Check sheet for the modelled part. Datum: model origin and axes. Units: mm. Face numbers are marked on the shaded views. A direction names the side the tool comes from. Coordinates: 2 decimals unless noted, no trailing zeros. Loops run counter-clockwise (first coordinate to the right, second up) from the corner with the lowest first, then second, coordinate; pieces in that order, holes last. Notation, with made-up numbers: (8.5, 48) -> (44.5, 48) arc R31 ccw to (44.5, 76) -> close; hole circle Ø7 at (-30.5, -17). An arc over 180 degrees is marked (long way). Use CSV: the item, a comma, the result in double quotes.
```python
from build123d import *

# Parameters (mm, degrees)
BOSS_EXTRUDE1_START = 0.2
BOSS_EXTRUDE1_DEPTH = 1
BOSS_EXTRUDE2_DEPTH = 0.2


with BuildPart() as part:
    # Sketch1 → Boss-Extrude1 (new body)
    with BuildSketch(Plane.XY.offset(BOSS_EXTRUDE1_START)):
        Polygon((-2.65, 2.65), (2.65, 2.65), (2.65, -1.15), (1.15, -2.65), (-1.15, -2.65), (-2.65, -1.15), align=None)
    extrude(amount=BOSS_EXTRUDE1_DEPTH)

    # Sketch2 → Revolve1 (revolve)
    with BuildSketch(Plane(origin=(0, 0, 0), x_dir=(0, 0, -1), z_dir=(1, 0, 0)), mode=Mode.PRIVATE) as revolve1_sk:
        with BuildLine():
            Line((-6, 0), (-6, 2.5))
            Line((-6, 2.5), (-2.2, 2.5))
            ThreePointArc((-2.2, 2.5), (-1.8, 2.1), (-1.4, 2.5))
            Line((-1.4, 2.5), (-1.2, 2.5))
            Line((-1.2, 2.5), (-1.2, 0))
            Line((-1.2, 0), (-6, 0))
        make_face()
    revolve(revolve1_sk.sketch.rotate(Axis((0, 0, 0), (0, 0, 1)), 90), axis=Axis((0, 0, 0), (0, 0, 1)))

    # Sketch3 → Boss-Extrude2 (add)
    with BuildSketch(Plane.XY):
        with BuildLine():
            Line((0.4, -1.1), (0.4, -3))
            Line((0.4, -3), (-0.4, -3))
            Line((-0.4, -3), (-0.4, -1.1))
            ThreePointArc((-0.4, -1.1), (0, -0.7), (0.4, -1.1))
        make_face()
    boss_extrude2 = extrude(amount=BOSS_EXTRUDE2_DEPTH)

    # Mirror1: Boss-Extrude2 across plane
    add(boss_extrude2.mirror(Plane.ZX))


solid = part.part
```
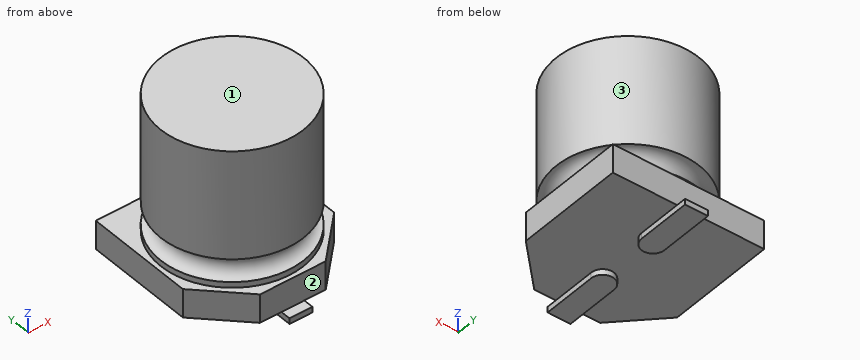
1) Cross-section at B-B on y = 0. Record the boundary of the cut face in (x, z).
Answer below:
outline,"(-2.65, 0.2) -> (2.65, 0.2) -> (2.65, 1.2) -> (2.5, 1.2) -> (2.5, 1.4) arc R0.4 cw to (2.5, 2.2) -> (2.5, 6) -> (-2.5, 6) -> (-2.5, 2.2) arc R0.4 cw to (-2.5, 1.4) -> (-2.5, 1.2) -> (-2.65, 1.2) -> close"
2) Thickness scan on line 1 along Z through (x, y) = (1.5, -2.05); line 2 along Z through (x, y) = (1, 0.05); line 3 along Z through (x, y) = (2.05, -1). Record the ranges inside material, lowest first. Write a range as from..to.
Answer below:
line 1,"z = 0.2..1.2"
line 2,"z = 0.2..6"
line 3,"z = 0.2..1.47, 2.13..6"
3) Access from +Z, -Z, +X, -X, +Y, -Y to the whole of each face (thin tool, end or side, straight path). Record for the marked faces 1, 2 and 3.
Answer below:
face 1,"+Z, +X, -X, +Y, -Y"
face 2,"+Z, +X, -X, -Y"
face 3,"+Z"
4) Go/stop test with flat-tipped pins: pin 1 Ø1 at (x, z) = (0, 1) entering from +Y; pin 2 Ø1.1 at (x, z) = (0, 1) entering from -Y. Record where each tip stops, or that it passes through.
Answer below:
pin 1,"stops at y = 2.65"
pin 2,"stops at y = -2.65"
5) Cross-section at C-C on z = 3.9. Record the boundary of the cut face in (x, y), and give its area (3 significant figures).
Answer below:
outline,"circle Ø5 at (0, 0)"
area,"19.6 mm²"
6) Cross-section at A-A on x = 0. Record the boundary of the cut face in (y, z), and give its area (3 significant figures).
Answer below:
outline,"(-3, 0) -> (-0.7, 0) -> (-0.7, 0.2) -> (0.7, 0.2) -> (0.7, 0) -> (3, 0) -> (3, 0.2) -> (2.65, 0.2) -> (2.65, 1.2) -> (2.5, 1.2) -> (2.5, 1.4) arc R0.4 cw to (2.5, 2.2) -> (2.5, 6) -> (-2.5, 6) -> (-2.5, 2.2) arc R0.4 cw to (-2.5, 1.4) -> (-2.5, 1.2) -> (-2.65, 1.2) -> (-2.65, 0.2) -> (-3, 0.2) -> close"
area,"29.7 mm²"
